Design review of the part built by this model. Coordinates are the model's own, in mm. Coordinates: 2 decimals unless noted, no trailing zeros. Write each loop counter-clockwise with the first axis right and the second up, starting at its lowest first coordinate (ties: lowest second). Pieces come first, ordered by that corner, then holes. Notation, with made-up numbers: M 56.25,-38 L 89.25,-38 A9 ccw 89.25,-33 Z; hole C -18,3 d5. An arc over 180 degrees is marked long. Write item = value, one per line.
```python
from build123d import *

# Parameters (mm, degrees)
SKETCH1_W           = 226
SKETCH1_H           = 223
SKETCH1_R           = 1.45
BOSS_EXTRUDE1_DEPTH = 6
SKETCH2_R           = 2
SKETCH2_R_2         = 9
SKETCH2_R_3         = 10
SKETCH2_W           = 25
SKETCH2_H           = 25
CUT_EXTRUDE1_DEPTH  = 7
FILLET1_R           = 5
FILLET2_R           = 2


with BuildPart() as part:
    # Sketch1 → Boss-Extrude1 (new body)
    with BuildSketch(Plane(origin=(0, 0, 0), x_dir=(1, 0, 0), z_dir=(0, 1, 0))):
        with Locations((0, -1.5)):
            Rectangle(SKETCH1_W, SKETCH1_H)
        with Locations((-95, -105)):
            Circle(SKETCH1_R, mode=Mode.SUBTRACT)
        with Locations((-95, 105)):
            Circle(SKETCH1_R, mode=Mode.SUBTRACT)
        with Locations((95, 105)):
            Circle(SKETCH1_R, mode=Mode.SUBTRACT)
        with Locations((95, -105)):
            Circle(SKETCH1_R, mode=Mode.SUBTRACT)
        Polygon((-5, -85.375), (0.5, -85.375), (0.5, -82.375), (7, -82.375), (7, -47.625), (0.5, -47.625), (0.5, -44.625), (-5, -44.625), align=None, mode=Mode.SUBTRACT)
        with BuildLine():
            Line((6, -12.5), (6, -22.5))
            ThreePointArc((6, -22.5), (-3, -31.5), (-12, -22.5))
            Line((-12, -22.5), (-12, -12.5))
            ThreePointArc((-12, -12.5), (-3, -3.5), (6, -12.5))
        make_face(mode=Mode.SUBTRACT)
    extrude(amount=BOSS_EXTRUDE1_DEPTH)

    # Sketch2 → Cut-Extrude1 (cut, through all)
    with BuildSketch(Plane(origin=(0, 6, 0), x_dir=(1, 0, 0), z_dir=(0, 1, 0))):
        with Locations((-28, -100.5)):
            Circle(SKETCH2_R)
        with Locations((22, -100.5)):
            Circle(SKETCH2_R)
        with Locations((-80, 88.5)):
            Circle(SKETCH2_R)
        with Locations((77, 84.5)):
            Circle(SKETCH2_R)
        with Locations((-93, 15.5)):
            Circle(SKETCH2_R)
        with Locations((52, 62.5)):
            Circle(SKETCH2_R)
        with Locations((-60, 67.5)):
            Circle(SKETCH2_R_2)
        with Locations((77, 62.5)):
            Circle(SKETCH2_R_3)
        with BuildLine():
            Line((90, -35), (90, -5))
            ThreePointArc((90, -5), (95, 0), (100, -5))
            Line((100, -5), (100, -35))
            ThreePointArc((100, -35), (95, -40), (90, -35))
        make_face()
        with Locations((49.5, 97.5)):
            Rectangle(SKETCH2_W, SKETCH2_H)
    extrude(amount=-CUT_EXTRUDE1_DEPTH, mode=Mode.SUBTRACT)

    # Fillet1
    fillet1_edges = [part.edges().sort_by_distance(p)[0] for p in [
        (62, 3, -85),
        (37, 3, -85),
    ]]
    fillet(fillet1_edges, radius=FILLET1_R)

    # Fillet2
    fillet2_edges = [part.edges().sort_by_distance(p)[0] for p in [
        (-113, 3, -110),
        (113, 3, -110),
        (113, 3, 113),
        (-113, 3, 113),
    ]]
    fillet(fillet2_edges, radius=FILLET2_R)


solid = part.part
```
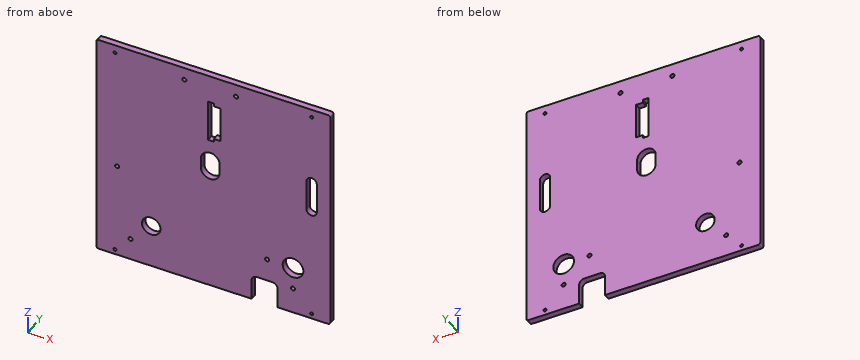
Q1. For P1, Ø1.8, axis at x = 46, y = 3, coming from the -Z side, flat-tipped, find the tip position at first contact; note if it passes through.
Check result:
P1 = -85
Q2. Consider section D-D, the plane y = 2.45. State how many separate pieces and enclosed holes the cut face has, and give its area (3 significant figures).
Check result:
separate_pieces = 1
enclosed_holes = 15
area = 47,800 mm²
Q3. Consider section B-B, the plane z = 8. State the section outline as (x, y) points.
Check result:
outline = M -113,0 L -10.79,0 L -10.79,6 L -113,6 Z; M 4.79,0 L 90,0 L 90,6 L 4.79,6 Z; M 100,0 L 113,0 L 113,6 L 100,6 Z
Q4. Wall thickness on line 1 (X direction, y = 4.7, z = 105); line 2 (X direction, y = 4.75, z = 100.5); line 3 (X direction, y = 2.4, z = -105): over which ranges is each line inside the solid? List them lowest first.
Check result:
line_1 = -113 to -96.45, -93.55 to 93.55, 96.45 to 113
line_2 = -113 to -30, -26 to 20, 24 to 113
line_3 = -113 to -96.45, -93.55 to 37, 62 to 93.55, 96.45 to 113
Q5. Consider section C-C, the plane x = -61. State the section outline as (y, z) points.
Check result:
outline = M 0,-110 L 6,-110 L 6,-76.44 L 0,-76.44 Z; M 0,-58.56 L 6,-58.56 L 6,113 L 0,113 Z
Q6. Consider section A-A, the plane z = 75.5. State the section outline as (x, y) points.
Check result:
outline = M -113,0 L -5,0 L -5,6 L -113,6 Z; M 7,0 L 113,0 L 113,6 L 7,6 Z
